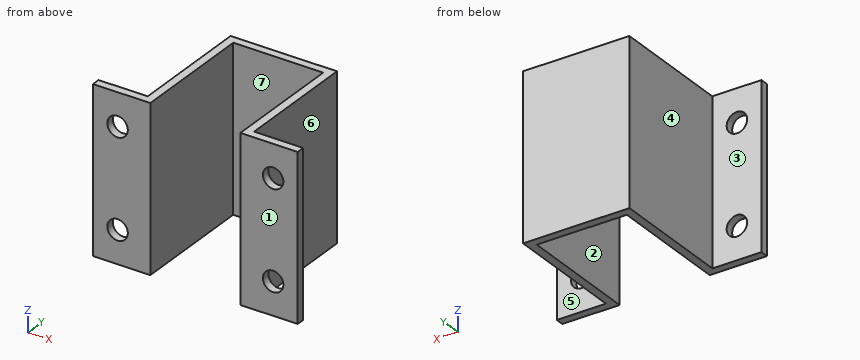
```python
from build123d import *

# Parameters (mm, degrees)
BOSS_EXTRUDE3_DEPTH = 50.8
CUT_EXTRUDE1_REACH  = 4.54
SKETCH6_R           = 3.175


with BuildPart() as part:
    # Sketch5 → Boss-Extrude3 (new body)
    with BuildSketch(Plane.XY):
        Polygon((0, 0), (17.78, 0), (17.78, 38.1), (31.75, 38.1), (31.75, 40.64), (15.24, 40.64), (15.24, 2.54), (0, 2.54), align=None)
    boss_extrude3 = extrude(amount=BOSS_EXTRUDE3_DEPTH)

    # Mirror6: Boss-Extrude3 across plane
    add(boss_extrude3.mirror(Plane(origin=(31.75, 40.64, 50.8), x_dir=(0, 0, 1), z_dir=(-1, 0, 0))))

    # Sketch6 → Cut-Extrude1 (cut, up to next)
    with BuildSketch(Plane(origin=(0, 2.54, 0), x_dir=(-1, 0, 0), z_dir=(0, 1, 0)), mode=Mode.PRIVATE) as cut_extrude1_sk1:
        with Locations((-7.62, 40.64)):
            Circle(SKETCH6_R)
    cut_extrude1_tool1 = extrude(cut_extrude1_sk1.sketch, amount=-CUT_EXTRUDE1_REACH, mode=Mode.PRIVATE) & part.part
    add(cut_extrude1_tool1.solids().sort_by_distance((7.62, 2.54, 40.64))[0], mode=Mode.SUBTRACT)
    # Sketch6 → Cut-Extrude1 (cut, up to next)
    with BuildSketch(Plane(origin=(0, 2.54, 0), x_dir=(-1, 0, 0), z_dir=(0, 1, 0)), mode=Mode.PRIVATE) as cut_extrude1_sk2:
        with Locations((-7.62, 10.16)):
            Circle(SKETCH6_R)
    cut_extrude1_tool2 = extrude(cut_extrude1_sk2.sketch, amount=-CUT_EXTRUDE1_REACH, mode=Mode.PRIVATE) & part.part
    add(cut_extrude1_tool2.solids().sort_by_distance((7.62, 2.54, 10.16))[0], mode=Mode.SUBTRACT)
    # Sketch6 → Cut-Extrude1 (cut, up to next)
    with BuildSketch(Plane(origin=(0, 2.54, 0), x_dir=(-1, 0, 0), z_dir=(0, 1, 0)), mode=Mode.PRIVATE) as cut_extrude1_sk3:
        with Locations((-55.88, 10.16)):
            Circle(SKETCH6_R)
    cut_extrude1_tool3 = extrude(cut_extrude1_sk3.sketch, amount=-CUT_EXTRUDE1_REACH, mode=Mode.PRIVATE) & part.part
    add(cut_extrude1_tool3.solids().sort_by_distance((55.88, 2.54, 10.16))[0], mode=Mode.SUBTRACT)
    # Sketch6 → Cut-Extrude1 (cut, up to next)
    with BuildSketch(Plane(origin=(0, 2.54, 0), x_dir=(-1, 0, 0), z_dir=(0, 1, 0)), mode=Mode.PRIVATE) as cut_extrude1_sk4:
        with Locations((-55.88, 40.64)):
            Circle(SKETCH6_R)
    cut_extrude1_tool4 = extrude(cut_extrude1_sk4.sketch, amount=-CUT_EXTRUDE1_REACH, mode=Mode.PRIVATE) & part.part
    add(cut_extrude1_tool4.solids().sort_by_distance((55.88, 2.54, 40.64))[0], mode=Mode.SUBTRACT)


solid = part.part
```
Geometry: final body of the model. Coordinates: model frame, mm. Face numbers are marked on the shaded views. A direction names the side the tool comes from. Coordinates: 2 decimals unless noted, no trailing zeros. Order: outer loops, then holes, each group sorted by start corner. A loop starts at its lowest first (then second) coordinate and runs counter-clockwise, first axis right, second up. Notation, with made-up numbers: M 86,78.5 L 139,78.5 A25 ccw 139,113.5 Z; hole C 75.25,53.5 d7. An arc over 180 degrees is marked long. Answer in a Markdown table with one row per item. Add a question column.
Q1. Line query: L1, parallel to X at y = 1, z = 10; L2, parallel to Z at x = 7.62, y = 1.3 (3 decimals); L3, parallel to X at y = 28.5, z = 30. Output: solid intervals per line, ascending.
Q2. Section query A-A on x = 7.62. Return the cut outline in (y, z) (3 decimals), and give its area (3 significant figures).
Q3. Contact query for flat-ended pins moving along their axis: P1, Ø4, axis at x = 54, z = 17, coming from the -Y side; P2, Ø2, axis at y = 7, z = 44, coming from the +X side; P3, Ø11.5, axis at y = 27, z = 18, coming from the -X side; P4, Ø8, axis at x = 38, z = 7, coming from the -Y side. Output: stop coordinate, or through.
Q4. Section query B-B on y = 10.5. Return the cut outline in (x, z), and give its area (3 significant figures).
Q5. Section query D-D on z = 29. Return the cut outline in (x, y), and give its area (3 significant figures).
Q6. Reachability of the marked faces 1, 2 and 3 from +Z, -Z, +X, -X, +Y, -Y: full face, straight path, thin tool, end or side. Return the list, or none.
Q7. Section query C-C on z = 10.16. Return the cut outline in (x, y) (3 decimals).
Q8. Mould query, pull axis X, two halves, no side actions, for the marked faces 4, 5, 6 and 7. Classes: released by +X, released by -X, zero draft, split by the parting line, or undercut.
Completed:
| question | item | result |
|---|---|---|
| 1 | L1 | x = 0 to 4.45, 10.79 to 17.78, 45.72 to 52.71, 59.05 to 63.5 |
| 1 | L2 | z = 0 to 6.985, 13.335 to 37.465, 43.815 to 50.8 |
| 1 | L3 | x = 15.24 to 17.78, 45.72 to 48.26 |
| 2 | outline | M 0,0 L 2.54,0 L 2.54,6.985 L 0,6.985 Z; M 0,13.335 L 2.54,13.335 L 2.54,37.465 L 0,37.465 Z; M 0,43.815 L 2.54,43.815 L 2.54,50.8 L 0,50.8 Z |
| 2 | area | 96.8 mm2 |
| 3 | P1 | stops at y = 0 |
| 3 | P2 | stops at x = 48.26 |
| 3 | P3 | stops at x = 15.24 |
| 3 | P4 | stops at y = 38.1 |
| 4 | outline | M 15.24,0 L 17.78,0 L 17.78,50.8 L 15.24,50.8 Z; M 45.72,0 L 48.26,0 L 48.26,50.8 L 45.72,50.8 Z |
| 4 | area | 258 mm2 |
| 5 | outline | M 0,0 L 17.78,0 L 17.78,38.1 L 45.72,38.1 L 45.72,0 L 63.5,0 L 63.5,2.54 L 48.26,2.54 L 48.26,40.64 L 15.24,40.64 L 15.24,2.54 L 0,2.54 Z |
| 5 | area | 355 mm2 |
| 6 | face 1 | +Z, -Z, +X, -X, -Y |
| 6 | face 2 | +Z, -Z, -Y |
| 6 | face 3 | +Z, -Z, -X, +Y |
| 7 | outline | M 0,0 L 4.445,0 L 4.445,2.54 L 0,2.54 Z; M 10.795,0 L 17.78,0 L 17.78,38.1 L 45.72,38.1 L 45.72,0 L 52.705,0 L 52.705,2.54 L 48.26,2.54 L 48.26,40.64 L 15.24,40.64 L 15.24,2.54 L 10.795,2.54 Z; M 59.055,0 L 63.5,0 L 63.5,2.54 L 59.055,2.54 Z |
| 8 | face 4 | released by -X |
| 8 | face 5 | zero draft |
| 8 | face 6 | released by +X |
| 8 | face 7 | undercut |
